Part model, mm, in its own coordinate system. Face numbers are marked on the shaded views. A direction names the side the tool comes from. Coordinates: 2 decimals unless noted, no trailing zeros. Write each loop counter-clockwise with the first axis right and the second up, starting at its lowest first coordinate (ties: lowest second). Pieces come first, ordered by that corner, then holes. Notation, with made-up numbers: (-0.75, 13) - (17.25, 13) arc R12 cw to (17.25, 25) - close; hole circle Ø1 at (-28.5, 55.25). An arc over 180 degrees is marked (long way). Use a Markdown table: item, result.
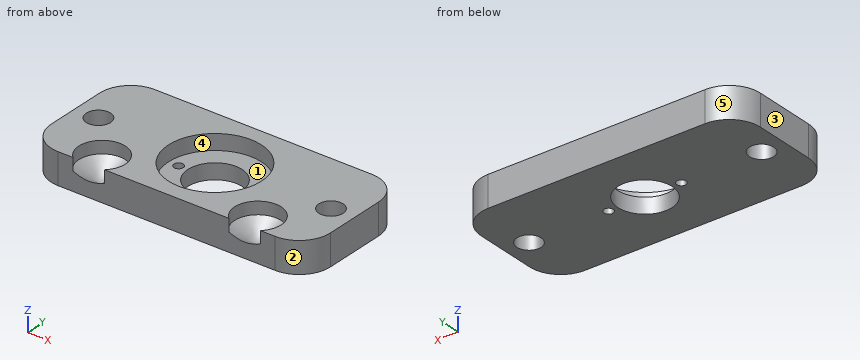
Autodesk Inventor part; units mm, degrees
ref_plane "YZ Plane" through (0, 0, 0) normal (1, 0, 0) x (0, 1, 0)
ref_plane "XZ Plane" through (0, 0, 0) normal (0, 1, 0) x (-1, 0, 0)
ref_plane "XY Plane" through (0, 0, 0) normal (0, 0, 1) x (1, 0, 0)
sketch "Sketch1" plane through (0, 0, 0) normal (0, 0, 1) x (1, 0, 0)
  line L0 (-28.575, -12.7) -> (28.575, -12.7)
  line L1 (28.575, -12.7) -> (28.575, 12.7)
  line L2 (28.575, 12.7) -> (-28.575, 12.7)
  line L3 (-28.575, 12.7) -> (-28.575, -12.7)
  point P0 (0, 0)
  dimension "d0" = 57.15
  dimension "d1" = 25.4
  dimension "d33" = 28.575
  dimension "d34" = 12.7
extrude "Extrusion1" add sketch "Sketch1" along normal blind 3.175 and the other way blind 3.175
sketch "Sketch2" plane through (0, 0, 3.175) normal (0, 0, 1) x (1, 0, 0)
  line L0 (-28.575, -12.7) -> (28.575, -12.7)
  line L1 (28.575, -12.7) -> (28.575, 12.7)
  line L2 (28.575, 12.7) -> (-28.575, 12.7)
  line L3 (-28.575, 12.7) -> (-28.575, -12.7)
  point P0 (0, 0)
  point P1 (0, 0)
  dimension "d4" = 28.575
  dimension "d5" = 12.7
  dimension "d6" = 57.15
hole "Hole1" at (0, 0, 3.175) direction (0, 0, -1) diameter 11.1125 end through all counterbore diameter 19.05 counterbore depth 3.175
sketch "Sketch3" plane through (0, 0, 3.175) normal (0, 0, 1) x (1, 0, 0)
  circle A0 centre (0, 0) radius 9.525
  line L0 (-28.575, -12.7) -> (28.575, -12.7)
  line L1 (28.575, -12.7) -> (28.575, 12.7)
  line L2 (28.575, 12.7) -> (-28.575, 12.7)
  line L3 (-28.575, 12.7) -> (-28.575, -12.7)
  point P0 (0, 0)
  point P1 (-23.8124, -0.0762)
  point P2 (23.8124, -0.0762)
  dimension "d14" = 23.8125
  dimension "d15" = 23.8125
  dimension "d59" = 0.0762
hole "Hole2" at (-23.8124, -0.0762, 3.175) at (23.8124, -0.0762, 3.175) direction (0, 0, -1) diameter 4.9784 end through all
sketch "Sketch4" plane through (0, 0, 3.175) normal (0, 0, 1) x (1, 0, 0)
  circle A0 centre (-23.8124, -0.0762) radius 2.4892
  circle A1 centre (23.8124, -0.0762) radius 2.4892
  circle A2 centre (0, 0) radius 9.525
  line L0 (-28.575, -12.7) -> (28.575, -12.7)
  line L1 (28.575, -12.7) -> (28.575, 12.7)
  line L2 (28.575, 12.7) -> (-28.575, 12.7)
  line L3 (-28.575, 12.7) -> (-28.575, -12.7)
  point P0 (0, 0)
  point P1 (-7.4422, 0)
  point P2 (7.4422, 0)
  dimension "d23" = 7.4422
  dimension "d24" = 7.4422
hole "Hole3" at (-7.4422, 0, 3.175) at (7.4422, 0, 3.175) direction (0, 0, -1) diameter 1.9304 end through all
fillet "Fillet1" radius 6.35 4 edges at (28.575, 12.7, 0) (-28.575, 12.7, 0) (-28.575, -12.7, 0) (28.575, -12.7, 0)
sketch "Sketch5" plane through (0, 0, 3.175) normal (0, 0, 1) x (1, 0, 0)
  line L0 (28.575, -6.35) -> (28.575, 6.35)
  line L1 (-28.575, 6.35) -> (-28.575, -6.35)
  line L2 (-22.225, -12.7) -> (22.225, -12.7)
  line L3 (22.225, 12.7) -> (-22.225, 12.7)
  point P0 (0, 0)
  point P1 (15.9512, -9.1948)
  point P2 (-15.9512, -9.1948)
  dimension "d41" = 12.6238
  dimension "d42" = 12.6238
  dimension "d43" = 3.5052
hole "Hole5" at (15.9512, -9.1948, 3.175) at (-15.9512, -9.1948, 3.175) direction (0, 0, -1) diameter 9.525 depth 2.54 tip angle 118
properties part number "CHA_010_EncoderMountRev0" material "ABS Plastic"
Item 1: Band-saw the part on D-D, the plane y = 0. Give the cut face in (x, z) (3 decimals).
From the geometry:
| item | result |
|---|---|
| outline | (-28.575, -3.175) - (-26.3, -3.175) - (-26.3, 3.175) - (-28.575, 3.175) - close; (-21.324, -3.175) - (-8.407, -3.175) - (-8.407, 0) - (-9.525, 0) - (-9.525, 3.175) - (-21.324, 3.175) - close; (-6.477, -3.175) - (-5.556, -3.175) - (-5.556, 0) - (-6.477, 0) - close; (5.556, -3.175) - (6.477, -3.175) - (6.477, 0) - (5.556, 0) - close; (8.407, -3.175) - (21.324, -3.175) - (21.324, 3.175) - (9.525, 3.175) - (9.525, 0) - (8.407, 0) - close; (26.3, -3.175) - (28.575, -3.175) - (28.575, 3.175) - (26.3, 3.175) - close |
Item 2: Band-saw the part on B-B, the plane y = 4.5. Give the cut face in (x, z) (3 decimals), then the cut area to 3 significant figures.
From the geometry:
| item | result |
|---|---|
| outline | (-28.575, -3.175) - (-3.259, -3.175) - (-3.259, 0) - (-8.395, 0) - (-8.395, 3.175) - (-28.575, 3.175) - close; (3.259, -3.175) - (28.575, -3.175) - (28.575, 3.175) - (8.395, 3.175) - (8.395, 0) - (3.259, 0) - close |
| area | 289 mm^2 |
Item 3: Band-saw the part on C-C, the plane z = 1.75. Count the separate pieces of the cut face and the enclosed holes in it, then the cut area to 3 significant figures.
From the geometry:
| item | result |
|---|---|
| separate pieces | 1 |
| enclosed holes | 3 |
| area | 962 mm^2 |
Item 4: Two-plate mould, pull along Y, no slides. Class the marked faces 1, 2 and 3: pulls with the +Y half, pulls with the -Y half, needs draft (parallel to the pull), parting line crosses it, or undercut.
From the geometry:
| item | result |
|---|---|
| face 1 | undercut |
| face 2 | pulls with the -Y half |
| face 3 | needs draft |
Item 5: Which spindle directions (+Z, -Z, +X, -X, +Y, -Y) get a long thin tool onto all of the face, cutting with end or side? Do the marked faces 4 and 5. Say none if no direction does.
From the geometry:
| item | result |
|---|---|
| face 4 | +Z |
| face 5 | +Z, -Z, -X, +Y |
Item 6: Drop flat-ended pins along their axis: P1, Ø5.5, axis at x = -23.81, y = -0.08, coming from the +Z side (3 decimals); P2, Ø3, axis at x = -7.44, y = 0, coming from the +Z side; P3, Ø9, axis at x = 0, y = 0, coming from the -Z side; P4, Ø5.5, axis at x = 15.95, y = -9.19, coming from the +Z side. Give the stop position or say it passes through.
From the geometry:
| item | result |
|---|---|
| P1 | z = 3.175 |
| P2 | z = 0 |
| P3 | through |
| P4 | z = -0.57 |
Item 7: Band-saw the part on A-A, the plane x = 0. Give the cut face in (y, z) (3 decimals).
From the geometry:
| item | result |
|---|---|
| outline | (-12.7, -3.175) - (-5.556, -3.175) - (-5.556, 0) - (-9.525, 0) - (-9.525, 3.175) - (-12.7, 3.175) - close; (5.556, -3.175) - (12.7, -3.175) - (12.7, 3.175) - (9.525, 3.175) - (9.525, 0) - (5.556, 0) - close |
Item 8: Drill centre lines: probe 1 along X at (y, z) = (0, -1.25) (3 decimals); probe 2 along Y at (x, z) = (0, -2.4); probe 3 along X at (y, z) = (-1.5, -0.5) (3 decimals). Where is each one in solid material? Low to high.
From the geometry:
| item | result |
|---|---|
| probe 1 | -28.575 to -26.3, -21.324 to -8.407, -6.477 to -5.556, 5.556 to 6.477, 8.407 to 21.324, 26.3 to 28.575 |
| probe 2 | -12.7 to -5.56, 5.56 to 12.7 |
| probe 3 | -28.575 to -25.854, -21.771 to -5.35, 5.35 to 21.771, 25.854 to 28.575 |
